Geometry check sheet. Reference: the model listing, model coordinates, mm. Round coordinates to 2 decimals unless told otherwise and drop trailing zeros. Loops run counter-clockwise (first coordinate to the right, second up) from the corner with the lowest first, then second, coordinate; pieces in that order, holes last. Notation, with made-up numbers: M 1,-14.5 L 39,-14.5 A20 cw 39,-2.5 Z; hole C 18.25,29.5 d5. An arc over 180 degrees is marked long. Use one line per item in the form item = value. Start each with the question number.
1. Cross-section at B-B (z = 186). Record the boundary of the cut face in (x, y), then the cut area to 3 significant figures.
2. Material ranges on line 1 (X direction, y = 0, z = 6.75); line 2 (Z direction, x = -0.25, y = -3.5), recorded low to high.
3. Cross-section at A-A (z = 268). Record the boundary of the cut face in (x, y), then the cut area to 3 significant figures.
4. Go/stop test with flat-tipped pins: pin 1 (13 mm diameter, centred on x = 3, z = 3, fed in from +Y); pin 2 (8 mm diameter, centred on y = -9.5, z = 235.5, fed in from -X) (3 decimals); pin 3 (14 mm diameter, centred on y = 0, z = 268, fed in from -X). Record where each tip stops, or that it passes through.
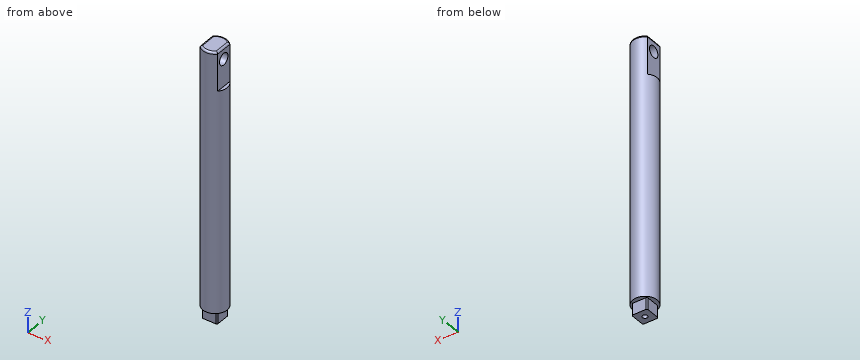
```python
from build123d import *

# Parameters (mm, degrees)
SKETCH1_R             = 12.5
BOSS_EXTRUDE1_DEPTH   = 280
CUT_EXTRUDE1_START    = -40
CUT_EXTRUDE1_DEPTH    = 40
SKETCH3_R             = 6
CUT_EXTRUDE2_DEPTH    = 282.102294548
FILLET1_R             = 2
SKETCH4_R             = 12.5
SKETCH4_W             = 16
SKETCH4_H             = 16
CUT_EXTRUDE3_DEPTH    = 12
M6_TAPPED_HOLE1_D     = 5
M6_TAPPED_HOLE1_DEPTH = 15
M6_TAPPED_HOLE1_TIP   = 1.502151548
CHAMFER1_SIZE         = 1


with BuildPart() as part:
    # Sketch1 → Boss-Extrude1 (new body)
    with BuildSketch(Plane.XY):
        Circle(SKETCH1_R)
    extrude(amount=BOSS_EXTRUDE1_DEPTH)

    # Sketch2 → Cut-Extrude1 (cut)
    with BuildSketch(Plane.XY.offset(280).offset(CUT_EXTRUDE1_START)):
        with BuildLine():
            Line((-9, -8.674675786), (-9, 8.674675786))
            ThreePointArc((-9, 8.674675786), (-12.5, 0), (-9, -8.674675786))
        make_face()
        with BuildLine():
            ThreePointArc((12.5, 0), (11.592023119, 4.677071733), (9, 8.674675786))
            Line((9, 8.674675786), (9, -8.674675786))
            ThreePointArc((9, -8.674675786), (11.592023119, -4.677071733), (12.5, 0))
        make_face()
    extrude(amount=CUT_EXTRUDE1_DEPTH, mode=Mode.SUBTRACT)

    # Sketch3 → Cut-Extrude2 (cut, through all)
    with BuildSketch(Plane.ZY.offset(9)):
        with Locations((268, 0)):
            Circle(SKETCH3_R)
    extrude(amount=-CUT_EXTRUDE2_DEPTH, mode=Mode.SUBTRACT)

    # Fillet1
    fillet1_edges = [part.edges().sort_by_distance(p)[0] for p in [
        (0, 12.5, 280),
        (9, 0, 280),
        (0, -12.5, 280),
        (-9, 0, 280),
    ]]
    fillet(fillet1_edges, radius=FILLET1_R)

    # Sketch4 → Cut-Extrude3 (cut)
    with BuildSketch(Plane(origin=(0, 0, 0), x_dir=(-1, 0, 0), z_dir=(0, 0, -1))):
        Circle(SKETCH4_R)
        Rectangle(SKETCH4_W, SKETCH4_H, mode=Mode.SUBTRACT)
    extrude(amount=-CUT_EXTRUDE3_DEPTH, mode=Mode.SUBTRACT)

    # M6 Tapped Hole1
    with Locations(Plane(origin=(0, 0, 0), x_dir=(-1, 0, 0), z_dir=(0, 0, -1))):
        with Locations((0, 0)):
            Hole(M6_TAPPED_HOLE1_D / 2, depth=M6_TAPPED_HOLE1_DEPTH)
            with Locations((0, 0, -(M6_TAPPED_HOLE1_DEPTH + M6_TAPPED_HOLE1_TIP / 2))):  # 118° drill point
                Cone(0, M6_TAPPED_HOLE1_D / 2, M6_TAPPED_HOLE1_TIP, mode=Mode.SUBTRACT)

    # Chamfer1
    chamfer1_edges = [part.edges().sort_by_distance(p)[0] for p in [
        (8, -8, 6),
        (-8, -8, 6),
        (-8, 8, 6),
        (8, 8, 6),
    ]]
    chamfer(chamfer1_edges, length=CHAMFER1_SIZE)


solid = part.part
```
Reported:
q1.outline = C 0,0 d25
q1.area = 491 mm²
q2.line_1 = -8 to -2.5, 2.5 to 8
q2.line_2 = 0 to 263.13, 272.87 to 280
q3.outline = M -9,-8.67 A12.5 ccw 9,-8.67 L 9,-6 L -9,-6 Z; M -9,6 L 9,6 L 9,8.67 A12.5 ccw -9,8.67 Z
q3.area = 191 mm²
q4.pin_1 = 8
q4.pin_2 = -11.225
q4.pin_3 = -9
